Read the model definition and answer for the solid it produces. Units are mm, in the model's axes. A direction names the side the tool comes from. Give positions to 0.01 mm unless a question says otherwise; leave off trailing zeros. Order: outer loops, then holes, each group sorted by start corner. A loop starts at its lowest first (then second) coordinate and runs counter-clockwise, first axis right, second up. Notation, with made-up numbers: M -28,-14.75 L -17,-14.75 A12 ccw -17,-9.75 Z; hole C 74.25,-38 d8. An arc over 180 degrees is marked long. One line per item, written item: value.
from build123d import *

# Parameters (mm, degrees)
EXTRU_MINCE1_DEPTH      = 128
ESQUISSE2_R             = 2.5
ENL_V_MAT_EXTRU_1_DEPTH = 10
ESQUISSE3_R             = 2.5
ESQUISSE3_W             = 18
ESQUISSE3_H             = 18.5
ENL_V_MAT_EXTRU_2_DEPTH = 10


with BuildPart() as part:
    # Esquisse1 → Extru.-Mince1 (new, symmetric)
    with BuildSketch(Plane(origin=(0, 0, 0), x_dir=(0, 0, -1), z_dir=(1, 0, 0))):
        Polygon((-20, 0), (0, 0), (0, -20), (-1.5, -20), (-1.5, -1.5), (-20, -1.5), align=None)
    extrude(amount=EXTRU_MINCE1_DEPTH, both=True)

    # Esquisse2 → Enlèv. mat.-Extru.1 (cut)
    with BuildSketch(Plane.XY.offset(1.5)):
        with Locations((-120, -10)):
            Circle(ESQUISSE2_R)
        with Locations(Location((120, -10, 0), (0, 0, 90))):
            Circle(ESQUISSE2_R)
    extrude(amount=-ENL_V_MAT_EXTRU_1_DEPTH, mode=Mode.SUBTRACT)

    # Esquisse3 → Enlèv. mat.-Extru.2 (cut)
    with BuildSketch(Plane.XZ.offset(1.5)):
        with Locations(Location((-38, 11.5, 0), (0, 0, 270))):
            Circle(ESQUISSE3_R)
        with Locations(Location((38, 11.5, 0), (0, 0, 90))):
            Circle(ESQUISSE3_R)
        with Locations((-119, 10.75)):
            Rectangle(ESQUISSE3_W, ESQUISSE3_H)
        with Locations((119, 10.75)):
            Rectangle(ESQUISSE3_W, ESQUISSE3_H)
    extrude(amount=-ENL_V_MAT_EXTRU_2_DEPTH, mode=Mode.SUBTRACT)


solid = part.part
1) Each of these flat-tipped pins is pushed along its axis until it touches: pin 1 Ø1.6 at (y, z) = (-0.5, 15.5) entering from +X; pin 2 Ø5.5 at (x, z) = (-7.5, 11) entering from -Y; pin 3 Ø5 at (x, y) = (-3, -6.5) entering from +Z; pin 4 Ø4 at (x, y) = (-120, -10) entering from -Z. Where does it stop, or does it pass through?
Reported:
pin 1: stops at x = 110
pin 2: stops at y = -1.5
pin 3: stops at z = 1.5
pin 4: passes through
2) Determine the mould class of faces 1 (the face through (2, -10, 0)), 2 (the face through (2, 0, 10)), 3 (the face through (-40.44, -0.76, 12.04)) for opening direction Z: +Z half, -Z half, draft (parallel to the pull), parting line (faces both ways), or undercut.
Reported:
face 1: -Z half
face 2: draft
face 3: undercut
3) Find section D-D, the plane x = -38. Write down the section's boundary in (y, z), plus the area to 4 significant figures.
Reported:
outline: M -20,0 L 0,0 L 0,9 L -1.5,9 L -1.5,1.5 L -20,1.5 Z; M -1.5,14 L 0,14 L 0,20 L -1.5,20 Z
area: 50.25 mm^2
4) Find section C-C, the plane y = -10. Write down the section's boundary in (x, z), plus the area to 3 significant figures.
Reported:
outline: M -128,0 L -122.5,0 L -122.5,1.5 L -128,1.5 Z; M -117.5,0 L 117.5,0 L 117.5,1.5 L -117.5,1.5 Z; M 122.5,0 L 128,0 L 128,1.5 L 122.5,1.5 Z
area: 369 mm^2
5) Consider probe 1 along Z at (x, y) = (38, -0.4); probe 2 along Y at (x, z) = (-120, 0.3); probe 3 along X at (y, z) = (-11, 1). Determine where each line is inside the solid, lowest interval first.
Reported:
probe 1: z = 0 to 9, 14 to 20
probe 2: y = -20 to -12.5, -7.5 to 0
probe 3: x = -128 to -122.29, -117.71 to 117.71, 122.29 to 128
6) Find section B-B, the plane x = -120. Write down the section's boundary in (y, z), plus the area to 3 significant figures.
Reported:
outline: M -20,0 L -12.5,0 L -12.5,1.5 L -20,1.5 Z; M -7.5,0 L 0,0 L 0,1.5 L -7.5,1.5 Z
area: 22.5 mm^2
7) Find section A-A, the plane z = 11.5. Write down the section's boundary in (x, y), plus the area to 3 significant figures.
Reported:
outline: M -110,-1.5 L -40.5,-1.5 L -40.5,0 L -110,0 Z; M -35.5,-1.5 L 35.5,-1.5 L 35.5,0 L -35.5,0 Z; M 40.5,-1.5 L 110,-1.5 L 110,0 L 40.5,0 Z
area: 315 mm^2
8) Which of the six approach directions +Z, -Z, +X, -X, +Y, -Y give full straight-line access (tool end or side, diameter ignored) to faces 4 (the face through (117.52, -10.33, 0.76)), 5 (the face through (2, -1.5, 11))?
Reported:
face 4: +Z, -Z
face 5: +Z, +X, -X, -Y
